from build123d import *

# Parameters (mm, degrees)
SKETCH1_W                 = 213
SKETCH1_H                 = 140.79
BOSS_EXTRUDE1_DEPTH       = 5
SKETCH2_W                 = 15
SKETCH2_H                 = 5
CUT_EXTRUDE1_DEPTH        = 128.760346059
CUT_EXTRUDE3_DEPTH        = 128.760346059
LPATTERN2_COUNT           = 4
LPATTERN2_PITCH           = 60
LPATTERN1_COUNT           = 7
LPATTERN1_PITCH           = 30
LPATTERN1_COPY_1_SKETCH_W = 15
LPATTERN1_COPY_1_SKETCH_H = 5
LPATTERN1_COPY_1_DEPTH    = 128.760346059
LPATTERN1_COPY_2_SKETCH_W = 15
LPATTERN1_COPY_2_SKETCH_H = 5
LPATTERN1_COPY_2_DEPTH    = 128.760346059
LPATTERN1_COPY_3_SKETCH_W = 15
LPATTERN1_COPY_3_SKETCH_H = 5
LPATTERN1_COPY_3_DEPTH    = 128.760346059
LPATTERN1_COPY_4_SKETCH_W = 15
LPATTERN1_COPY_4_SKETCH_H = 5
LPATTERN1_COPY_4_DEPTH    = 128.760346059
LPATTERN1_COPY_5_SKETCH_W = 15
LPATTERN1_COPY_5_SKETCH_H = 5
LPATTERN1_COPY_5_DEPTH    = 128.760346059
LPATTERN1_COPY_6_SKETCH_W = 15
LPATTERN1_COPY_6_SKETCH_H = 5
LPATTERN1_COPY_6_DEPTH    = 128.760346059
SKETCH3_W                 = 5
SKETCH3_H                 = 15
SKETCH3_W_2               = 15
SKETCH3_H_2               = 5
CUT_EXTRUDE2_DEPTH        = 128.760346059
MIRROR2_COPY_1_DEPTH      = 128.760346059
MIRROR2_COPY_2_DEPTH      = 128.760346059
MIRROR2_COPY_3_DEPTH      = 128.760346059
CUT_EXTRUDE4_DEPTH        = 128.760346059
SKETCH7_W                 = 3
SKETCH7_H                 = 5
CUT_EXTRUDE5_DEPTH        = 128.760346059


with BuildPart() as part:
    # Sketch1 → Boss-Extrude1 (new body)
    with BuildSketch(Plane(origin=(0, 0, 0), x_dir=(1, 0, 0), z_dir=(0, 1, 0))):
        Rectangle(SKETCH1_W, SKETCH1_H)
    extrude(amount=BOSS_EXTRUDE1_DEPTH)

    # Sketch2 → Cut-Extrude1 (cut, through all)
    with BuildSketch(Plane.XZ):
        with Locations((99, 67.895)):
            Rectangle(SKETCH2_W, SKETCH2_H)
    cut_extrude1 = extrude(amount=-CUT_EXTRUDE1_DEPTH, mode=Mode.SUBTRACT)

    # Sketch5 → Cut-Extrude3 (cut, through all)
    with BuildSketch(Plane.XZ):
        with BuildLine():
            Line((100.5, 59.395), (97.5, 59.395))
            ThreePointArc((97.5, 59.395), (96.5, 60.395), (97.5, 61.395))
            Line((97.5, 61.395), (100.5, 61.395))
            ThreePointArc((100.5, 61.395), (101.5, 60.395), (100.5, 59.395))
        make_face()
    cut_extrude3 = extrude(amount=-CUT_EXTRUDE3_DEPTH, mode=Mode.SUBTRACT)

    # LPattern2: Cut-Extrude3 ×4
    with Locations(*[(-i * LPATTERN2_PITCH, 0, 0) for i in range(1, LPATTERN2_COUNT)]):
        add(cut_extrude3, mode=Mode.SUBTRACT)

    # Mirror1: Cut-Extrude1 across plane
    add(cut_extrude1.mirror(Plane.XY), mode=Mode.SUBTRACT)

    # LPattern1: Cut-Extrude1 ×7
    with Locations(*[(-i * LPATTERN1_PITCH, 0, 0) for i in range(1, LPATTERN1_COUNT)]):
        add(cut_extrude1, mode=Mode.SUBTRACT)

    # LPattern1 copy 1 sketch → LPattern1 copy 1 (cut, through all)
    with BuildSketch(Plane(origin=(-30, 0, 0), x_dir=(1, 0, 0), z_dir=(0, -1, 0))):
        with Locations((99, -67.895)):
            Rectangle(LPATTERN1_COPY_1_SKETCH_W, LPATTERN1_COPY_1_SKETCH_H)
    extrude(amount=-LPATTERN1_COPY_1_DEPTH, mode=Mode.SUBTRACT)

    # LPattern1 copy 2 sketch → LPattern1 copy 2 (cut, through all)
    with BuildSketch(Plane(origin=(-60, 0, 0), x_dir=(1, 0, 0), z_dir=(0, -1, 0))):
        with Locations((99, -67.895)):
            Rectangle(LPATTERN1_COPY_2_SKETCH_W, LPATTERN1_COPY_2_SKETCH_H)
    extrude(amount=-LPATTERN1_COPY_2_DEPTH, mode=Mode.SUBTRACT)

    # LPattern1 copy 3 sketch → LPattern1 copy 3 (cut, through all)
    with BuildSketch(Plane(origin=(-90, 0, 0), x_dir=(1, 0, 0), z_dir=(0, -1, 0))):
        with Locations((99, -67.895)):
            Rectangle(LPATTERN1_COPY_3_SKETCH_W, LPATTERN1_COPY_3_SKETCH_H)
    extrude(amount=-LPATTERN1_COPY_3_DEPTH, mode=Mode.SUBTRACT)

    # LPattern1 copy 4 sketch → LPattern1 copy 4 (cut, through all)
    with BuildSketch(Plane(origin=(-120, 0, 0), x_dir=(1, 0, 0), z_dir=(0, -1, 0))):
        with Locations((99, -67.895)):
            Rectangle(LPATTERN1_COPY_4_SKETCH_W, LPATTERN1_COPY_4_SKETCH_H)
    extrude(amount=-LPATTERN1_COPY_4_DEPTH, mode=Mode.SUBTRACT)

    # LPattern1 copy 5 sketch → LPattern1 copy 5 (cut, through all)
    with BuildSketch(Plane(origin=(-150, 0, 0), x_dir=(1, 0, 0), z_dir=(0, -1, 0))):
        with Locations((99, -67.895)):
            Rectangle(LPATTERN1_COPY_5_SKETCH_W, LPATTERN1_COPY_5_SKETCH_H)
    extrude(amount=-LPATTERN1_COPY_5_DEPTH, mode=Mode.SUBTRACT)

    # LPattern1 copy 6 sketch → LPattern1 copy 6 (cut, through all)
    with BuildSketch(Plane(origin=(-180, 0, 0), x_dir=(1, 0, 0), z_dir=(0, -1, 0))):
        with Locations((99, -67.895)):
            Rectangle(LPATTERN1_COPY_6_SKETCH_W, LPATTERN1_COPY_6_SKETCH_H)
    extrude(amount=-LPATTERN1_COPY_6_DEPTH, mode=Mode.SUBTRACT)

    # Sketch3 → Cut-Extrude2 (cut, through all)
    with BuildSketch(Plane.XZ):
        with Locations((-1, 47.895)):
            Rectangle(SKETCH3_W, SKETCH3_H)
        with Locations((-1, -47.895)):
            Rectangle(SKETCH3_W, SKETCH3_H)
        with Locations((84, -47.895)):
            Rectangle(SKETCH3_W, SKETCH3_H)
        with Locations((84, 47.895)):
            Rectangle(SKETCH3_W, SKETCH3_H)
        with Locations((-91, 13)):
            Rectangle(SKETCH3_W_2, SKETCH3_H_2)
        with Locations((-91, -13)):
            Rectangle(SKETCH3_W_2, SKETCH3_H_2)
    extrude(amount=-CUT_EXTRUDE2_DEPTH, mode=Mode.SUBTRACT)

    # Mirror2: Cut-Extrude3 across plane
    add(cut_extrude3.mirror(Plane.XY), mode=Mode.SUBTRACT)

    # Mirror2 copy 1 sketch → Mirror2 copy 1 (cut, through all)
    with BuildSketch(Plane(origin=(-60, 0, 0), x_dir=(1, 0, 0), z_dir=(0, -1, 0))):
        with BuildLine():
            Line((100.5, -59.395), (97.5, -59.395))
            ThreePointArc((97.5, -59.395), (96.5, -60.395), (97.5, -61.395))
            Line((97.5, -61.395), (100.5, -61.395))
            ThreePointArc((100.5, -61.395), (101.5, -60.395), (100.5, -59.395))
        make_face()
    extrude(amount=-MIRROR2_COPY_1_DEPTH, mode=Mode.SUBTRACT)

    # Mirror2 copy 2 sketch → Mirror2 copy 2 (cut, through all)
    with BuildSketch(Plane(origin=(-120, 0, 0), x_dir=(1, 0, 0), z_dir=(0, -1, 0))):
        with BuildLine():
            Line((100.5, -59.395), (97.5, -59.395))
            ThreePointArc((97.5, -59.395), (96.5, -60.395), (97.5, -61.395))
            Line((97.5, -61.395), (100.5, -61.395))
            ThreePointArc((100.5, -61.395), (101.5, -60.395), (100.5, -59.395))
        make_face()
    extrude(amount=-MIRROR2_COPY_2_DEPTH, mode=Mode.SUBTRACT)

    # Mirror2 copy 3 sketch → Mirror2 copy 3 (cut, through all)
    with BuildSketch(Plane(origin=(-180, 0, 0), x_dir=(1, 0, 0), z_dir=(0, -1, 0))):
        with BuildLine():
            Line((100.5, -59.395), (97.5, -59.395))
            ThreePointArc((97.5, -59.395), (96.5, -60.395), (97.5, -61.395))
            Line((97.5, -61.395), (100.5, -61.395))
            ThreePointArc((100.5, -61.395), (101.5, -60.395), (100.5, -59.395))
        make_face()
    extrude(amount=-MIRROR2_COPY_3_DEPTH, mode=Mode.SUBTRACT)

    # Sketch6 → Cut-Extrude4 (cut, through all)
    with BuildSketch(Plane.XZ):
        with BuildLine():
            Line((-92.5, 22.5), (-89.5, 22.5))
            ThreePointArc((-89.5, 22.5), (-88.5, 21.5), (-89.5, 20.5))
            Line((-89.5, 20.5), (-92.5, 20.5))
            ThreePointArc((-92.5, 20.5), (-93.5, 21.5), (-92.5, 22.5))
        make_face()
        with BuildLine():
            Line((-92.5, -22.5), (-89.5, -22.5))
            ThreePointArc((-89.5, -22.5), (-88.5, -21.5), (-89.5, -20.5))
            Line((-89.5, -20.5), (-92.5, -20.5))
            ThreePointArc((-92.5, -20.5), (-93.5, -21.5), (-92.5, -22.5))
        make_face()
    extrude(amount=-CUT_EXTRUDE4_DEPTH, mode=Mode.SUBTRACT)

    # Sketch7 → Cut-Extrude5 (cut, through all)
    with BuildSketch(Plane.XZ):
        with Locations((-105, 67.895)):
            Rectangle(SKETCH7_W, SKETCH7_H)
        with Locations((-105, -67.895)):
            Rectangle(SKETCH7_W, SKETCH7_H)
    extrude(amount=-CUT_EXTRUDE5_DEPTH, mode=Mode.SUBTRACT)


solid = part.part
Geometry check sheet. Reference: the model listing, model coordinates, mm. A direction names the side the tool comes from. Give positions to 0.01 mm unless a question says otherwise; leave off trailing zeros. Order: outer loops, then holes, each group sorted by start corner. A loop starts at its lowest first (then second) coordinate and runs counter-clockwise, first axis right, second up.
1. Access from +Z, -Z, +X, -X, +Y, -Y to the whole of each face (thin tool, end or side, straight path). Record for faces 4 (the face through (84, 2, 70.395)), 5 (the face through (-91, 2, 10.5)), 6 (the face through (76.5, 2, -68)), 7 (the face through (76.5, 2, 68)), 8 (the face through (-66, 2, -70.395)).
Completed:
face 4: +Z, +X, -X, +Y, -Y
face 5: +Y, -Y
face 6: -Z, +Y, -Y
face 7: +Z, +Y, -Y
face 8: -Z, +X, -X, +Y, -Y
2. Sectioned sample at B-B (x = 68.5). Record the boundary of the cut face in (y, z) (3 decimals), then the cut area to 3 significant figures.
Completed:
outline: (0, -65.395) - (5, -65.395) - (5, 65.395) - (0, 65.395) - close
area: 654 mm2
3. Sectioned sample at A-A (y = 3.1). State how many separate pieces and enclosed holes the cut face has, then the cut area to 3 significant figures.
Completed:
separate pieces: 1
enclosed holes: 16
area: 28,400 mm2
4. Depth check by flat-ended pin: pin 1 (2.5 mm diameter, centred on x = 39.5, y = 2.5, fed in from -Z) (3 decimals); pin 2 (2.5 mm diameter, centred on x = -87.5, y = 3.5, fed in from -Z) (3 decimals); pin 3 (2.5 mm diameter, centred on x = 39, y = 3.5, fed in from +Z) (3 decimals); pin 4 (1.5 mm diameter, centred on y = 2, z = -68.5, fed in from -X). Enter the tip coordinate at first touch or a pass-through.
Completed:
pin 1: stops at z = -65.395
pin 2: stops at z = -70.395
pin 3: stops at z = 65.395
pin 4: stops at x = -103.5
5. Draft check along X on faces 1 (the face through (61.5, 2, 68)), 2 (the face through (-66, 2, 70.395)), 3 (the face through (106.5, 2, 1)). Enter one of: pulls with the +X half, pulls with the -X half, needs draft (parallel to the pull), parting line crosses it, or undercut.
Completed:
face 1: undercut
face 2: needs draft
face 3: pulls with the +X half
6. Scan lines: line 1 (Z direction, x = -80, y = 1.65) (3 decimals); line 2 (X direction, y = 0.6, z = -42); line 3 (Z direction, x = -98, y = 0.65) (3 decimals). Record each from-to range of solid material in increasing order.
Completed:
line 1: z = -65.395 to -61.395, -59.395 to 59.395, 61.395 to 65.395
line 2: x = -106.5 to -3.5, 1.5 to 81.5, 86.5 to 106.5
line 3: z = -70.395 to -15.5, -10.5 to 10.5, 15.5 to 70.395
